Part model, mm, in its own coordinate system. A direction names the side the tool comes from. Coordinates: 2 decimals unless noted, no trailing zeros. Order: outer loops, then holes, each group sorted by start corner. A loop starts at its lowest first (then second) coordinate and runs counter-clockwise, first axis right, second up.
1) Wall check: L1, parallel to Z at x = 0, y = 129.75; L2, parallel to Z at x = 0, y = 120.5; L3, parallel to Y at x = -3, z = -10.25. Give the ranges that are in metal, low to high.
2) Mould opens along Z. For faces 1 (the conical face through (0.2, 24.8, 11.7)), 2 (the conical face through (-0.22, 105.35, 0.53)), 3 (the cylindrical face through (-1.172, 79.723, 8.923)), 4 (the cylindrical face through (1.27, 121.79, 3.07)) say: +Z half, -Z half, draft (parallel to the pull), parting line (faces both ways), or undercut.
3) Cut at A-A (y = -106). List the corners of the cut face in (x, z).
4) Pin check, flat tips, straight feed: pin 1 Ø6 at (x, y) = (-1, 83.5) entering from -Z; pin 2 Ø1.5 at (x, y) = (1.5, 83.5) entering from -Z; pin 3 Ø2.5 at (x, z) = (-11.5, -3) entering from +Y. Stop position of each tip, or through.
5) Tool access for faces 5 (the flat face through (-9, -160, 5)), 6 (the flat face through (5, 25, 8)), 7 (the flat face through (9.5, 21, 0)): list every direction of +Z, -Z, +X, -X, +Y, -Y with a clear straight run to the whole face (end or side of a thin tool).
6) Cut at B-B (y = 35). List the corners of the cut face in (x, z), and give its area (3 significant figures).
Autodesk Inventor part; units mm, degrees
ref_plane "YZ Plane" through (0, 0, 0) normal (1, 0, 0) x (0, 1, 0)
ref_plane "XZ Plane" through (0, 0, 0) normal (0, 1, 0) x (-1, 0, 0)
sketch "Эскиз1" plane through (0, 0, 0) normal (0, 0, 1) x (1, 0, 0)
  line L0 (0, 137) -> (0, -200)
  line L1 (0, 137) -> (9, 137)
  line L2 (9, 137) -> (9, 25)
  line L3 (9, 25) -> (12.5, 25)
  line L4 (12.5, 25) -> (12.5, -180)
  line L5 (12.5, -180) -> (0, -180)
  line L6 (10, -180) -> (10, -160)
  line L7 (10, -160) -> (12.5, -160)
  point P0 (0, 0)
  point P1 (0, -177.0364)
  dimension "d1" = 200
  dimension "d2" = 18
  dimension "d3" = 25
  dimension "d7" = 25
  dimension "d8" = 137
  dimension "d16" = 180
  dimension "d17" = 20
  dimension "d18" = 20
revolve "Вращение1" add sketch "Эскиз1" angle 360 about axis through (0, 137, 0) along (0, -1, 0) contours L1 L2 L3 L4 L7 L6 L5 L0
sketch "Эскиз2" plane through (0, 137, 0) normal (0, 1, 0) x (1, 0, 0)
  point P0 (0, 0)
hole "Отверстие1" at (0, 137, 0) direction (0, -1, 0) diameter 6.647 depth 30 tip angle 118
thread "Резьба1"
ref_plane "РабПлоскость1" through (0, 81, -9) normal (0, 0, 1) x (1, 0, 0)
sketch "Эскиз3" plane through (0, 81, -9) normal (0, 0, 1) x (1, 0, 0)
  line L0 (0, 46) -> (0, -24) construction
  line L1 (-2.55, 46) -> (-2.55, -24)
  line L2 (2.55, -24) -> (2.55, 46)
  arc A0 (2.55, 46) -> (-2.55, 46) centre (0, 46) ccw
  arc A1 (-2.55, -24) -> (2.55, -24) centre (0, -24) ccw
  line L3 (-9, 56) -> (9, 56)
  point P0 (0, -81)
  point P1 (0, 11)
  point P2 (0, 56)
  dimension "d21" = 10
  dimension "d22" = 70
  dimension "d23" = 5.1
extrude "Выдавливание1" cut sketch "Эскиз3" along normal blind 2
chamfer "Chamfer1" distance 1 angle 45 4 edges at (-9, 137, 0) (-12.5, 25, 0) (-12.5, -160, 0) (-10, -180, 0)
sketch "Sketch4" plane through (0, 0, 0) normal (0, 0, 1) x (1, 0, 0)
  line L0 (12.5, 24) -> (-12.5, 24)
  line L1 (-12.5, -159) -> (12.5, -159)
  line L2 (-11.5, 25) -> (11.5, 25)
  line L3 (12.5, 24) -> (-12.5, 24)
  line L4 (-11.5, 25) -> (11.5, 25)
  line L5 (9.5, 25) -> (9.5, 17)
  line L6 (9.5, 17) -> (12.5, 17)
  line L7 (-12.5, 17) -> (-9.5, 17)
  line L8 (-9.5, 17) -> (-9.5, 25)
  line L9 (-9, 25) -> (9, 25)
  line L10 (0, 25) -> (0, 9.8425) construction
  line L11 (12.5, 24) -> (-12.5, 24)
  line L12 (12.5, 24) -> (12.5, 17)
  line L13 (11.5, 25) -> (12.5, 24)
  line L14 (11.5, 25) -> (12.5, 24)
  line L15 (-11.5, 25) -> (-12.5, 24)
  line L16 (-11.5, 25) -> (-12.5, 24)
  line L17 (-12.5, 17) -> (-12.5, 24)
  line L18 (-12.5, 24) -> (-12.5, -159)
  point P0 (0, 0)
  dimension "d29" = 19
  dimension "d30" = 8
extrude "Extrusion2" cut sketch "Sketch4" along normal through all both and the other way through all contours L12 L6 L5 L0 | L0 L5 L2 L13 | L8 L7 L17 L0 | L0 L15 L2 L8
properties part number "Вал"
Geometry check:
1. L1: z = -9 to -3.32, 3.32 to 9
1. L2: z = -7 to -3.32, 3.32 to 9
1. L3: y = -160 to 25
2. face 1: +Z half
2. face 2: undercut
2. face 3: parting line
2. face 4: undercut
3. outline: circle Ø25 at (0, 0)
4. pin 1: stops at z = -8.63
4. pin 2: stops at z = -7
4. pin 3: stops at y = 17
5. face 5: -Y
5. face 6: +Y
5. face 7: +Z, -Z, +X, +Y
6. outline: circle Ø18 at (0, 0)
6. area: 254 mm2
